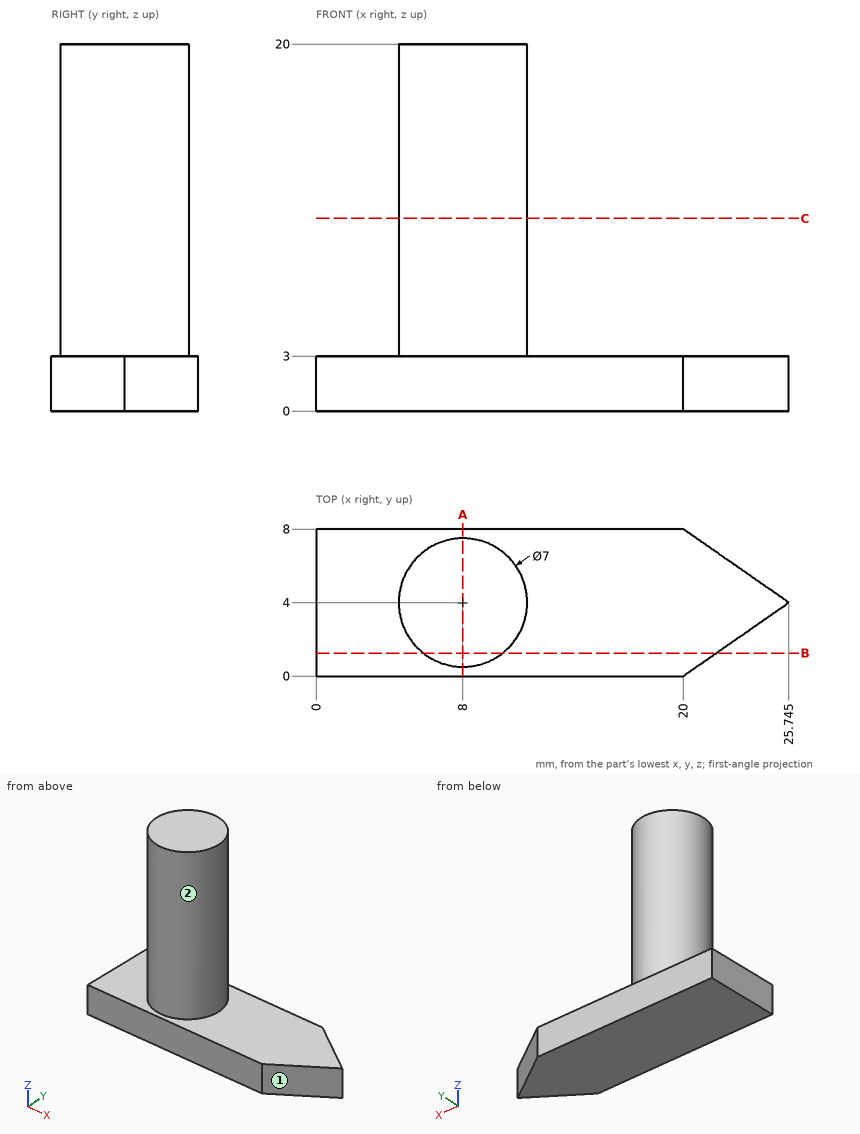
Study the drawing (mm; zero at the part's minimum x, y, z) and answer. A direction names the side the tool comes from. Give positions to 0.01 mm unless a question says otherwise; leave off trailing zeros. Order: outer loops, then holes, each group sorted by start corner. A loop starts at its lowest first (then second) coordinate and runs counter-clockwise, first axis right, second up. Notation, with made-up numbers: (-29.5, 27) -> (15.5, 27) arc R29 cw to (15.5, 65) -> close; hole circle Ø1 at (13.5, 67.25). An arc over 180 degrees is marked (long way). Put each result on its own line as item: value.
Item 1: A cutting plane is placed at A-A on x = 8. Give the vertices of the cut face in (y, z), plus the area to 3 significant figures.
Established:
outline: (0, 0) -> (8, 0) -> (8, 3) -> (7.5, 3) -> (7.5, 20) -> (0.5, 20) -> (0.5, 3) -> (0, 3) -> close
area: 143 mm^2
Item 2: Straight lines are drawn through the part: line 1 (Z direction, x = 3.5, y = 3.25); line 2 (X direction, y = 1.5, z = 1.5) (1 decimal); line 3 (X direction, y = 5, z = 17.75) (1 decimal). For each, find the intervals that lie inside material, in ascending order.
Established:
line 1: z = 0 to 3
line 2: x = 0 to 22.2
line 3: x = 4.6 to 11.4
Item 3: For the marked faces 1 and 2, determine the directions among +Z, -Z, +X, -X, +Y, -Y from which every point of the face is accessible in a straight line to the end or side of a thin tool.
Established:
face 1: +Z, -Z, +X, -Y
face 2: +Z
Item 4: Given P1, Ø3, axis at x = 7.5, z = 17, coming from the +Y side; P2, Ø1, axis at x = 5.5, z = 10, coming from the +Y side; P3, Ø4, axis at x = 17.5, y = 3.5, coming from the +Z side, each flat-ended and moving along its own axis, determine where each tip first touches the part or whether it passes through.
Established:
P1: stops at y = 7.5
P2: stops at y = 6.87
P3: stops at z = 3
Item 5: A cutting plane is placed at C-C on z = 10.5. Give the vertices of the cut face in (x, y), plus the area to 3 significant figures.
Established:
outline: circle Ø7 at (8, 4)
area: 38.5 mm^2
Item 6: A cutting plane is placed at B-B on y = 1.25. Give the vertices of the cut face in (x, z) (1 decimal), plus the area to 3 significant figures.
Established:
outline: (0, 0) -> (21.8, 0) -> (21.8, 3) -> (10.2, 3) -> (10.2, 20) -> (5.8, 20) -> (5.8, 3) -> (0, 3) -> close
area: 139 mm^2
